Could you check a few things on this model? Use its own coordinates, in mm. Face numbers are marked on the shaded views. A direction names the side the tool comes from. Give positions to 0.01 mm unless a question says otherwise; leave off trailing zeros. Loops run counter-clockwise (first coordinate to the right, second up) from the corner with the lowest first, then second, coordinate; pieces in that order, holes last. Notation, with made-up numbers: (-15.5, 23) - (-0.5, 23) arc R27 ccw to (-0.5, 40) - close; hole circle Ø7 at (-2.75, -4.75). An arc over 180 degrees is marked (long way). One line per item, written item: value. Start each with the question number.
Q1. I want a section at A-A (z = -28.5). Please give me the cut outline in (x, y), then the cut area to 3 significant figures.
Q2. I want a section at B-B (z = -20). Please give me the cut outline in (x, y).
Q3. For the marked faces 1 and 2, which set-ups out of +Z, -Z, +X, -X, +Y, -Y let a thin tool reach every point of the face, with its end or its side?
Q4. I'm going to push flat-ended pins straight in: P1, Ø1.1, axis at x = -2.5, z = -9.5, coming from the +Y side; P2, Ø0.5, axis at x = -2.5, y = 0.5, coming from the -Z side; P3, Ø0.8, axis at y = 0.5, z = -10, coming from the -X side. Where does each tip first touch, or does it pass through?
Q5. If I drill on line 1 (X direction, y = -1, z = -28.5); line 2 (Z direction, x = -2.2, y = -0.4); line 3 (Y direction, x = -0.25, z = -29.5), over which ranges is the centre line in solid material (lowest first)? Write a range as from..to.
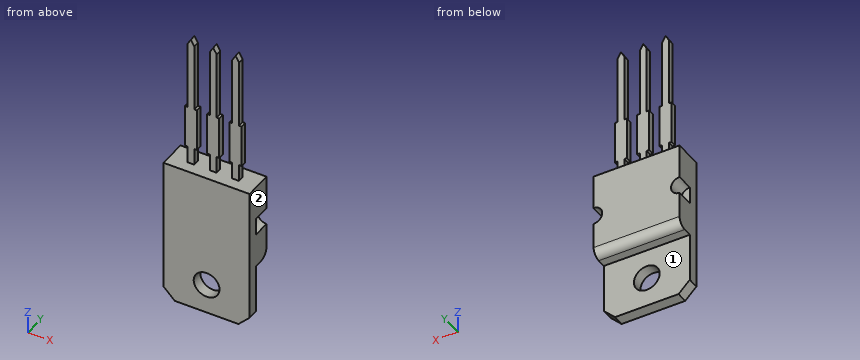
```python
from build123d import *

# Parameters (mm, degrees)
BOSS_EXTRUDE1_DEPTH   = 0.7
BOSS_EXTRUDE1_2_DEPTH = 0.7
BOSS_EXTRUDE1_3_DEPTH = 0.7
SKETCH2_W             = 10
SKETCH2_H             = 10
BOSS_EXTRUDE2_DEPTH   = 2
FILLET1_R             = 1
SKETCH3_R             = 1
CUT_EXTRUDE1_DEPTH    = 2
BOSS_EXTRUDE3_DEPTH   = 1.3
SKETCH5_R             = 1.5
CUT_EXTRUDE2_DEPTH    = 2.3


with BuildPart() as part:
    # Sketch1 → Boss-Extrude1 (new body)
    with BuildSketch(Plane(origin=(0, 0, 0), x_dir=(1, 0, 0), z_dir=(0, 1, 0))):
        Polygon((0, 0), (0, 8), (-0.3, 8), (-0.3, 13), (0, 13), (0, 15), (0.8, 15), (0.8, 13), (1.1, 13), (1.1, 8), (0.8, 8), (0.8, 0), (0.4, -0.692820323), align=None)
    extrude(amount=BOSS_EXTRUDE1_DEPTH)



with BuildPart() as body_2:
    # Sketch1 → Boss-Extrude1 2 (new body)
    with BuildSketch(Plane(origin=(0, 0, 0), x_dir=(1, 0, 0), z_dir=(0, 1, 0))):
        Polygon((-1.8, 15), (-2.6, 15), (-2.6, 13), (-2.9, 13), (-2.9, 8), (-2.6, 8), (-2.6, 0), (-2.2, -0.692820323), (-1.8, 0), (-1.8, 8), (-1.5, 8), (-1.5, 13), (-1.8, 13), align=None)
    extrude(amount=BOSS_EXTRUDE1_2_DEPTH)


with BuildPart() as body_3:
    # Sketch1 → Boss-Extrude1 3 (new body)
    with BuildSketch(Plane(origin=(0, 0, 0), x_dir=(1, 0, 0), z_dir=(0, 1, 0))):
        Polygon((-5.5, 13), (-5.5, 8), (-5.2, 8), (-5.2, 0), (-4.8, -0.692820323), (-4.4, 0), (-4.4, 8), (-4.1, 8), (-4.1, 13), (-4.4, 13), (-4.4, 15), (-5.2, 15), (-5.2, 13), align=None)
    extrude(amount=BOSS_EXTRUDE1_3_DEPTH)


with BuildPart() as part_1:
    add(part.part)

    add(body_2.part)  # Boss-Extrude2 merges body 2

    add(body_3.part)  # Boss-Extrude2 merges body 3
    # Sketch2 → Boss-Extrude2 (add)
    with BuildSketch(Plane(origin=(0, 0, 0), x_dir=(1, 0, 0), z_dir=(0, 1, 0))):
        with Locations((-2.2, 20)):
            Rectangle(SKETCH2_W, SKETCH2_H)
    extrude(amount=BOSS_EXTRUDE2_DEPTH)

    # Fillet1
    fillet1_edges = [part_1.edges().sort_by_distance(p)[0] for p in [
        (-2.2, 2, -25),
    ]]
    fillet(fillet1_edges, radius=FILLET1_R)

    # Sketch3 → Cut-Extrude1 (cut)
    with BuildSketch(Plane(origin=(0, 2, 0), x_dir=(1, 0, 0), z_dir=(0, 1, 0))):
        with Locations((-7.2, 20)):
            Circle(SKETCH3_R)
        with Locations((2.8, 20)):
            Circle(SKETCH3_R)
    extrude(amount=-CUT_EXTRUDE1_DEPTH, mode=Mode.SUBTRACT)

    # Sketch4 → Boss-Extrude3 (add)
    with BuildSketch(Plane.XZ):
        Polygon((-7.2, -30.7), (-5.9, -32), (1.5, -32), (2.8, -30.7), (2.8, -15), (-7.2, -15), align=None)
    extrude(amount=BOSS_EXTRUDE3_DEPTH)

    # Sketch5 → Cut-Extrude2 (cut, through all)
    with BuildSketch(Plane(origin=(0, 0, 0), x_dir=(1, 0, 0), z_dir=(0, 1, 0))):
        with Locations((-2.2, 28.5)):
            Circle(SKETCH5_R)
    extrude(amount=-CUT_EXTRUDE2_DEPTH, mode=Mode.SUBTRACT)


solid = part_1.part
```
Worked answers:
1. outline: (-7.2, -1.3) - (-3.7, -1.3) - (-3.7, 0) - (-7.2, 0) - close; (-0.7, -1.3) - (2.8, -1.3) - (2.8, 0) - (-0.7, 0) - close
1. area: 9.10 mm²
2. outline: (-7.2, -1.3) - (2.8, -1.3) - (2.8, 0) - (1.8, 0) - (1.8, 2) - (-6.2, 2) - (-6.2, 0) - (-7.2, 0) - close
3. face 1: -Z, +X, -X, +Y
3. face 2: +Z, -Z, +X, +Y, -Y
4. P1: stops at y = 0.7
4. P2: stops at z = -25
4. P3: stops at x = -5.5
5. line 1: x = -7.2..-3.7, -0.7..2.8
5. line 2: z = -32..-30, -27..-15
5. line 3: y = -1.3..0
